Answer from the drawing. Dimensions are ordinates in mm from the lowest x, y and z of the part. A direction names the side the tool comes from. Round coordinates to 2 decimals unless told otherwise and drop trailing zeros. Write each loop counter-clockwise with the first axis right and the second up, starting at its lowest first coordinate (ties: lowest second). Pieces come first, ordered by that corner, then holes. Notation, with made-up numbers: M -26.5,2 L 7.5,2 A16 ccw 7.5,8 Z; hole C 85.5,59 d9. An arc over 180 degrees is marked long. Answer as CSV lines item,"result". Start each with the question number.
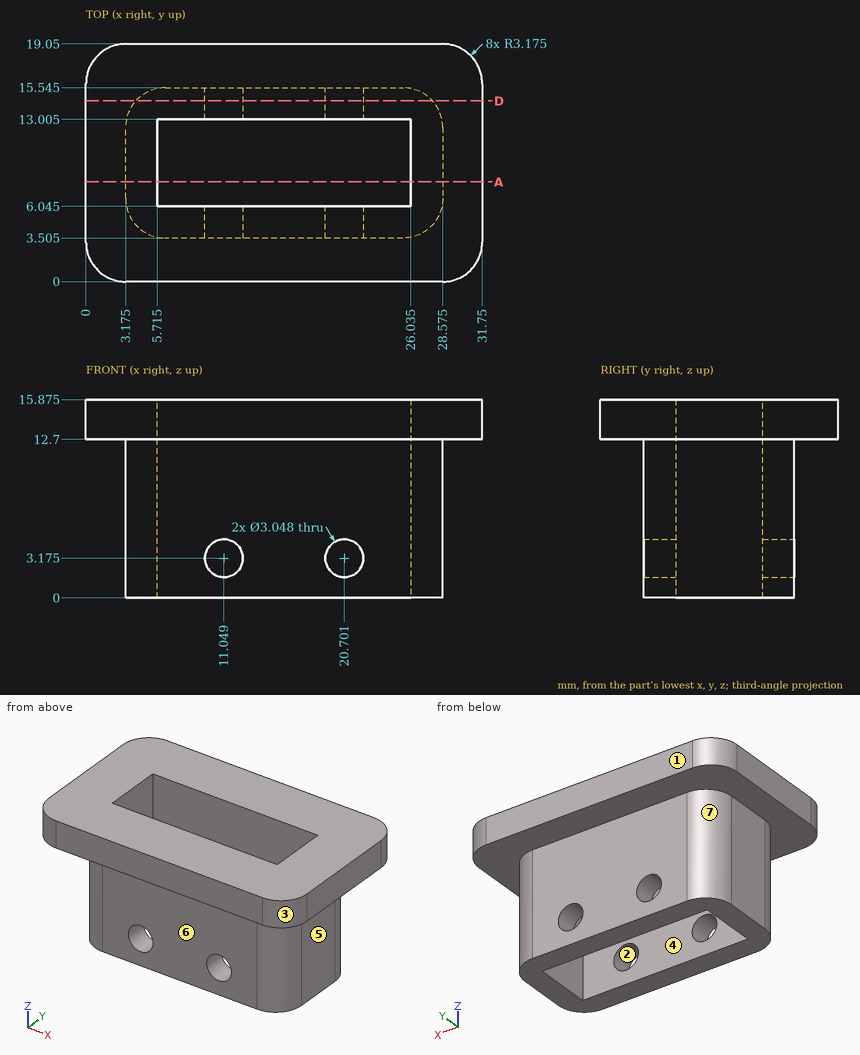
Q1. The mould has two halves that part along X. Classify the marked faces 1, 2 and 3: +X half, -X half, draft (parallel to the pull), parting line (faces both ways), or undercut.
Q2. Straight lines are drawn through the part: L1, parallel to X at y = 8.25, z = 12 (3 decimals); L2, parallel to Y at x = 13.5, z = 12.5 (1 decimal); L3, parallel to X at y = 11, z = 15 (3 decimals). For each, find the intervals that lie inside material, in ascending order.
Q3. For the marked faces 4, 5, 6 and 7, determine the directions among +Z, -Z, +X, -X, +Y, -Y from which every point of the face is accessible in a straight line to the end or side of a thin tool.
Q4. Find section A-A (y = 8). Determine the outline of the cut face in (x, z) (3 decimals).
Q5. Find section D-D (y = 14.5). Count the separate pieces of the cut face and the enclosed holes in it, plus the area to 3 significant figures.
Q6. Each of these flat-tipped pins is pushed along its axis until it touches: P1, Ø4, axis at x = 11.049, z = 3.175, coming from the -Y side (3 decimals); P2, Ø3.5, axis at y = 10, z = 5.5, coming from the -X side (3 decimals); P3, Ø5, axis at y = 5.5, z = 9, coming from the +X side (3 decimals); P4, Ø8, axis at x = 15, z = 10.5, coming from the +Y side. Where does it stop, or does it pass through?
Reported:
1,face 1,"draft"
1,face 2,"undercut"
1,face 3,"+X half"
2,L1,"x = 3.175 to 5.715, 26.035 to 28.575"
2,L2,"y = 3.5 to 6, 13 to 15.5"
2,L3,"x = 0 to 5.715, 26.035 to 31.75"
3,face 4,"+Z, -Z"
3,face 5,"-Z, +X, +Y, -Y"
3,face 6,"-Z, +X, -X, -Y"
3,face 7,"-Z, -X, +Y"
4,outline,"M 0,12.7 L 3.175,12.7 L 3.175,0 L 5.715,0 L 5.715,15.875 L 0,15.875 Z; M 26.035,0 L 28.575,0 L 28.575,12.7 L 31.75,12.7 L 31.75,15.875 L 26.035,15.875 Z"
5,separate pieces,"1"
5,enclosed holes,"2"
5,area,"388 mm2"
6,P1,"stops at y = 3.505"
6,P2,"stops at x = 3.175"
6,P3,"stops at x = 28.575"
6,P4,"stops at y = 19.05"
